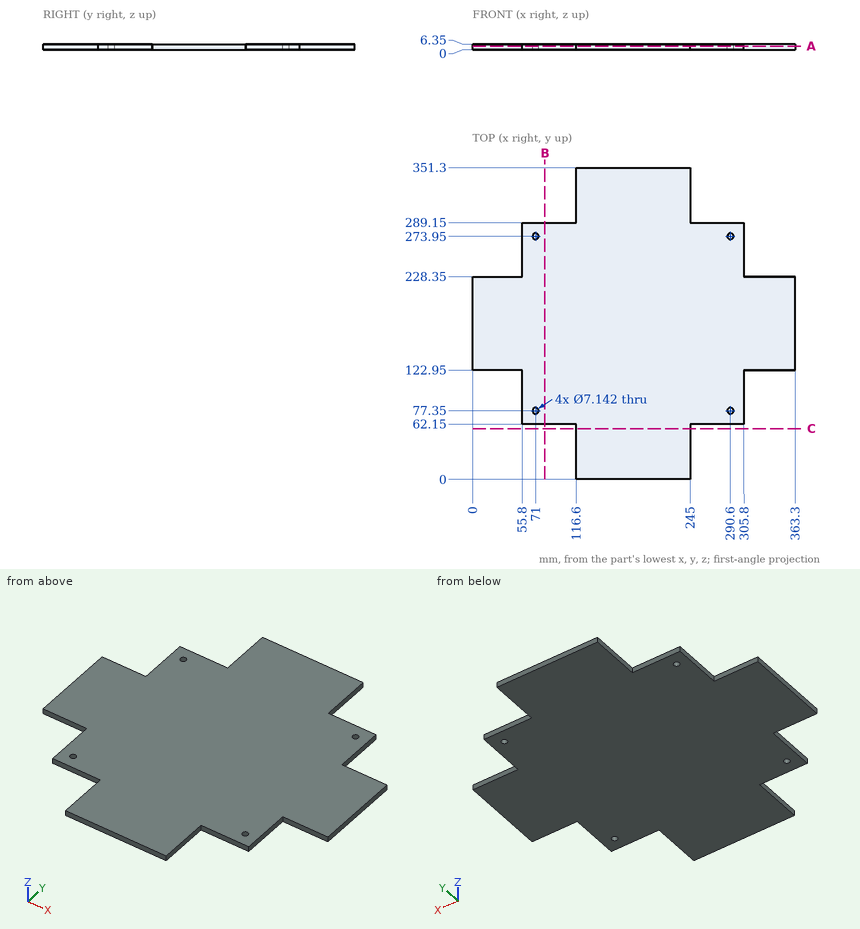
For this review, use the dimensioned drawing (mm, ordinates from the lowest corner) and the shaded views. Round coordinates to 2 decimals unless told otherwise and drop trailing zeros. Write each loop counter-clockwise with the first axis right and the second up, starting at its lowest first coordinate (ties: lowest second). Pieces come first, ordered by that corner, then holes. Notation, with made-up numbers: (-8.5, -7) -> (47.5, -7) arc R15 ccw to (47.5, -2) -> close; hole circle Ø8 at (52, 66). An arc over 180 degrees is marked (long way). One line per item, written item: value. Start each with the question number.
Q1. Insertion check: P1, Ø3, axis at x = 45.5, z = 4.5, coming from the -Y side; P2, Ø3, axis at y = 266, z = 4, coming from the -X side; P3, Ø1.9, axis at y = 311.5, z = 4.5, coming from the -X side; P4, Ø9.5, axis at x = 290.6, y = 273.95, coming from the +Z side. Each pin has a flat end and moves straight along its axis. Give the tip position at first contact, or say it passes through.
Q2. Add section A-A (z = 4). Give the boundary of the cut face in (x, y).
Q3. Add section B-B (x = 81.5). Give the boundary of the cut face in (y, z).
Q4. To check wall thickness, follow probe 1 along Y at (x, z) = (290.6, 4.5); probe 2 along X at (y, z) = (273.95, 4); probe 3 along Y at (x, z) = (340, 2.75). State the ranges of each line that lie inside material, in increasing order.
Q5. Add section C-C (y = 57). Give the boundary of the cut face in (x, z).
Response:
1. P1: stops at y = 122.95
1. P2: stops at x = 55.8
1. P3: stops at x = 116.6
1. P4: stops at z = 6.35
2. outline: (0, 122.95) -> (55.8, 122.95) -> (55.8, 62.15) -> (116.6, 62.15) -> (116.6, 0) -> (245, 0) -> (245, 62.15) -> (305.8, 62.15) -> (305.8, 122.95) -> (363.3, 122.95) -> (363.3, 228.35) -> (305.8, 228.35) -> (305.8, 289.15) -> (245, 289.15) -> (245, 351.3) -> (116.6, 351.3) -> (116.6, 289.15) -> (55.8, 289.15) -> (55.8, 228.35) -> (0, 228.35) -> close; hole circle Ø7.14 at (71, 77.35); hole circle Ø7.14 at (71, 273.95); hole circle Ø7.14 at (290.6, 77.35); hole circle Ø7.14 at (290.6, 273.95)
3. outline: (62.15, 0) -> (289.15, 0) -> (289.15, 6.35) -> (62.15, 6.35) -> close
4. probe 1: y = 62.15 to 73.78, 80.92 to 270.38, 277.52 to 289.15
4. probe 2: x = 55.8 to 67.43, 74.57 to 287.03, 294.17 to 305.8
4. probe 3: y = 122.95 to 228.35
5. outline: (116.6, 0) -> (245, 0) -> (245, 6.35) -> (116.6, 6.35) -> close
